from build123d import *

# Parameters (mm, degrees)
OUTER_CUT_DEPTH   = 1.5875
SLOTS_DEPTH       = 194.153806913
SKETCH3_R         = 1.5875
MOUNT_HOLES_DEPTH = 194.153806913


with BuildPart() as part:
    # Sketch1 → Outer Cut (new, symmetric)
    with BuildSketch(Plane(origin=(0, 0, 0), x_dir=(0, 0, -1), z_dir=(1, 0, 0))):
        with BuildLine():
            Line((-184.15, -31.75), (184.15, -31.75))
            ThreePointArc((184.15, -31.75), (188.640128061, -29.890128061), (190.5, -25.4))
            Line((190.5, -25.4), (190.5, 25.4))
            ThreePointArc((190.5, 25.4), (188.640128061, 29.890128061), (184.15, 31.75))
            Line((184.15, 31.75), (-184.15, 31.75))
            ThreePointArc((-184.15, 31.75), (-188.640128061, 29.890128061), (-190.5, 25.4))
            Line((-190.5, 25.4), (-190.5, -25.4))
            ThreePointArc((-190.5, -25.4), (-188.640128061, -29.890128061), (-184.15, -31.75))
        make_face()
    extrude(amount=OUTER_CUT_DEPTH, both=True)

    # Sketch2 → Slots (cut, through all)
    with BuildSketch(Plane(origin=(1.5875, 0, 0), x_dir=(0, 0, -1), z_dir=(1, 0, 0))):
        with BuildLine():
            Line((-177.8, 15.875), (177.8, 15.875))
            ThreePointArc((177.8, 15.875), (180.975, 12.7), (177.8, 9.525))
            Line((177.8, 9.525), (-177.8, 9.525))
            ThreePointArc((-177.8, 9.525), (-180.975, 12.7), (-177.8, 15.875))
        make_face()
        with BuildLine():
            Line((-177.8, -15.875), (177.8, -15.875))
            ThreePointArc((177.8, -15.875), (180.975, -12.7), (177.8, -9.525))
            Line((177.8, -9.525), (-177.8, -9.525))
            ThreePointArc((-177.8, -9.525), (-180.975, -12.7), (-177.8, -15.875))
        make_face()
    extrude(amount=-SLOTS_DEPTH, mode=Mode.SUBTRACT)

    # Sketch3 → Mount Holes (cut, through all)
    with BuildSketch(Plane(origin=(1.5875, 0, 0), x_dir=(0, 0, -1), z_dir=(1, 0, 0))):
        with Locations((-184.15, 25.4)):
            Circle(SKETCH3_R)
        with Locations((-174.625, 25.4)):
            Circle(SKETCH3_R)
        with Locations(Location((-174.625, -25.4, 0), (0, 0, 180))):
            Circle(SKETCH3_R)
        with Locations(Location((-184.15, -25.4, 0), (0, 0, 180))):
            Circle(SKETCH3_R)
        with Locations(Location((174.625, 25.4, 0), (0, 0, 180))):
            Circle(SKETCH3_R)
        with Locations(Location((184.15, 25.4, 0), (0, 0, 180))):
            Circle(SKETCH3_R)
        with Locations((184.15, -25.4)):
            Circle(SKETCH3_R)
        with Locations((174.625, -25.4)):
            Circle(SKETCH3_R)
    extrude(amount=-MOUNT_HOLES_DEPTH, mode=Mode.SUBTRACT)


solid = part.part
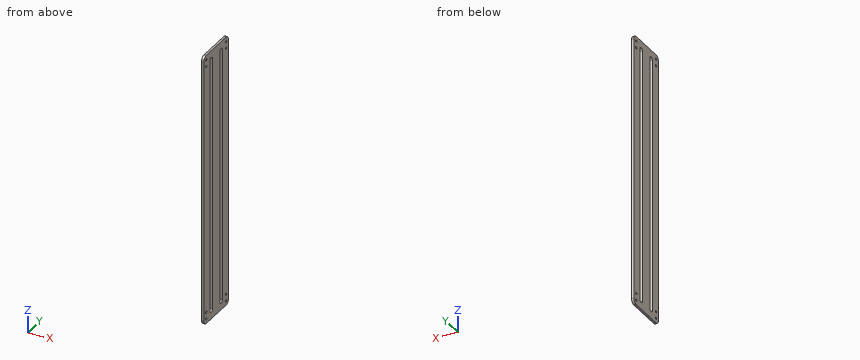
Can you work these out from the model? Positions are in its coordinate system, mm. Round coordinates to 2 decimals unless told otherwise and drop trailing zeros. Write each loop counter-clockwise with the first axis right and the second up, starting at its lowest first coordinate (ties: lowest second). Pieces come first, ordered by that corner, then holes. Notation, with made-up numbers: (49.5, 35) -> (59.5, 35) arc R31 cw to (59.5, 68) -> close; hole circle Ø3 at (82.5, 77.25). An arc over 180 degrees is marked (long way). Use one line per item in the form item = value. Start each with the question number.
Q1. I'm going to push a flat-ended pin straight in: P1, Ø5, axis at y = 25.4, z = 184.15, coming from the -X side. Where does the tip first touch, or does it pass through?
Q2. If I drill on probe 1 along Y at (x, z) = (0.2, -102.5) (3 decimals); probe 2 along Y at (x, z) = (-0.8, -184.15); probe 3 along Z at (x, y) = (0.1, -25), over which ranges is the centre line in solid material (lowest first)? Write a range as [from, to].
Q3. Imagine slicing it at B-B (x = 0.7). Count the separate pieces of the cut face and the enclosed holes in it, then the cut area to 3 significant figures.
Q4. Imagine slicing it at A-A (y = 12.7). Please give me the cut outline in (x, z) (1 decimal).
Worked out:
q1.P1 = -1.59
q2.probe_1 = [-31.75, -15.875], [-9.525, 9.525], [15.875, 31.75]
q2.probe_2 = [-31.75, -26.99], [-23.81, 23.81], [26.99, 31.75]
q2.probe_3 = [-190.5, -185.69], [-182.61, -176.16], [-173.09, 173.09], [176.16, 182.61], [185.69, 190.5]
q3.separate_pieces = 1
q3.enclosed_holes = 10
q3.area = 19,500 mm^2
q4.outline = (-1.6, -190.5) -> (1.6, -190.5) -> (1.6, -181) -> (-1.6, -181) -> close; (-1.6, 181) -> (1.6, 181) -> (1.6, 190.5) -> (-1.6, 190.5) -> close
